```python
from build123d import *

# Parameters (mm, degrees)
BOSS_EXTRUDE1_DEPTH = 17.78
SKETCH2_R           = 2.286
CUT_EXTRUDE1_DEPTH  = 36.070400967
SKETCH3_R           = 2.286
SKETCH3_R_2         = 4.572
CUT_EXTRUDE2_DEPTH  = 2.54
FILLET1_R           = 1.016
FILLET2_R           = 2.54


with BuildPart() as part:
    # Sketch1 → Boss-Extrude1 (new body)
    with BuildSketch(Plane(origin=(0, 0, 0), x_dir=(0, 0, -1), z_dir=(1, 0, 0))):
        Polygon((0, 0), (0, 27.432), (-12.7, 27.432), (-12.7, 15.24), (-3.556, 15.24), (-3.556, 0), align=None)
    extrude(amount=BOSS_EXTRUDE1_DEPTH)

    # Sketch2 → Cut-Extrude1 (cut, through all)
    with BuildSketch(Plane.XY.offset(12.7)):
        with Locations((4.445, 21.082)):
            Circle(SKETCH2_R)
        with Locations(Location((13.335, 21.082, 0), (0, 0, 180))):
            Circle(SKETCH2_R)
    extrude(amount=-CUT_EXTRUDE1_DEPTH, mode=Mode.SUBTRACT)

    # Sketch3 → Cut-Extrude2 (cut)
    # profile 1 of 4: a face of its own
    with BuildSketch(Plane.XY.offset(12.7)):
        with BuildLine():
            ThreePointArc((8.89, 20.011878979), (8.763, 21.082), (8.89, 22.152121021))
            ThreePointArc((8.89, 22.152121021), (4.445, 25.654), (0, 22.152121021))
            Line((0, 22.152121021), (0, 20.011878979))
            ThreePointArc((0, 20.011878979), (4.445, 16.51), (8.89, 20.011878979))
        make_face()
        with Locations((4.445, 21.082)):
            Circle(SKETCH3_R, mode=Mode.SUBTRACT)
    # profile 2 of 4: a face of its own
    with BuildSketch(Plane.XY.offset(12.7)):
        with BuildLine():
            ThreePointArc((8.89, 22.152121021), (8.985138985, 21.620815367), (9.017, 21.082))
            ThreePointArc((9.017, 21.082), (8.985138985, 20.543184633), (8.89, 20.011878979))
            ThreePointArc((8.89, 20.011878979), (13.335, 16.51), (17.78, 20.011878979))
            Line((17.78, 20.011878979), (17.78, 22.152121021))
            ThreePointArc((17.78, 22.152121021), (13.335, 25.654), (8.89, 22.152121021))
        make_face()
        with Locations((13.335, 21.082)):
            Circle(SKETCH3_R, mode=Mode.SUBTRACT)
    # profile 3 of 4: a face of its own
    with BuildSketch(Plane.XY.offset(12.7)):
        with Locations((4.445, 21.082)):
            Circle(SKETCH3_R_2)
    # profile 4 of 4: a face of its own
    with BuildSketch(Plane.XY.offset(12.7)):
        with Locations((13.335, 21.082)):
            Circle(SKETCH3_R_2)
    extrude(amount=-CUT_EXTRUDE2_DEPTH, mode=Mode.SUBTRACT)

    # Fillet1
    fillet1_edges = [part.edges().sort_by_distance(p)[0] for p in [
        (17.78, 15.24, 8.128),
        (8.89, 20.011878979, 11.43),
        (0, 20.011878979, 11.43),
        (0, 22.152121021, 11.43),
        (8.89, 22.152121021, 11.43),
        (17.78, 22.152121021, 11.43),
        (17.78, 20.011878979, 11.43),
        (0, 15.24, 8.128),
    ]]
    fillet(fillet1_edges, radius=FILLET1_R)

    # Fillet2
    # the kernel refuses this fillet: 2.54 mm, written as the material it takes off along each edge
    with BuildSketch(Plane(origin=(0, 27.432, -6.35), x_dir=(0, -1, 0), z_dir=(0, 0, 1))) as fillet2_piece_1:
        with BuildLine():
            CenterArc((FILLET2_R, FILLET2_R), FILLET2_R, 180, 90)
            Line((0, FILLET2_R), (-FILLET2_R * 0.02, FILLET2_R))
            Line((-FILLET2_R * 0.02, FILLET2_R), (-FILLET2_R * 0.02, -FILLET2_R * 0.02))
            Line((-FILLET2_R * 0.02, -FILLET2_R * 0.02), (FILLET2_R, -FILLET2_R * 0.02))
            Line((FILLET2_R, -FILLET2_R * 0.02), (FILLET2_R, 0))
        make_face()
    extrude(amount=25.4, mode=Mode.SUBTRACT)
    with BuildSketch(Plane(origin=(17.78, 27.432, -6.35), x_dir=(0, -1, 0), z_dir=(0, 0, 1))) as fillet2_piece_2:
        with BuildLine():
            CenterArc((FILLET2_R, -FILLET2_R), FILLET2_R, 90, 90)
            Line((0, -FILLET2_R), (-FILLET2_R * 0.02, -FILLET2_R))
            Line((-FILLET2_R * 0.02, -FILLET2_R), (-FILLET2_R * 0.02, FILLET2_R * 0.02))
            Line((-FILLET2_R * 0.02, FILLET2_R * 0.02), (FILLET2_R, FILLET2_R * 0.02))
            Line((FILLET2_R, FILLET2_R * 0.02), (FILLET2_R, 0))
        make_face()
    extrude(amount=25.4, mode=Mode.SUBTRACT)
    with BuildSketch(Plane(origin=(0, 0, 9.906), x_dir=(0, 1, 0), z_dir=(0, 0, -1))) as fillet2_piece_3:
        with BuildLine():
            CenterArc((FILLET2_R, FILLET2_R), FILLET2_R, 180, 90)
            Line((0, FILLET2_R), (-FILLET2_R * 0.02, FILLET2_R))
            Line((-FILLET2_R * 0.02, FILLET2_R), (-FILLET2_R * 0.02, -FILLET2_R * 0.02))
            Line((-FILLET2_R * 0.02, -FILLET2_R * 0.02), (FILLET2_R, -FILLET2_R * 0.02))
            Line((FILLET2_R, -FILLET2_R * 0.02), (FILLET2_R, 0))
        make_face()
    extrude(amount=16.256, mode=Mode.SUBTRACT)
    with BuildSketch(Plane(origin=(17.78, 0, 9.906), x_dir=(0, 1, 0), z_dir=(0, 0, -1))) as fillet2_piece_4:
        with BuildLine():
            CenterArc((FILLET2_R, -FILLET2_R), FILLET2_R, 90, 90)
            Line((0, -FILLET2_R), (-FILLET2_R * 0.02, -FILLET2_R))
            Line((-FILLET2_R * 0.02, -FILLET2_R), (-FILLET2_R * 0.02, FILLET2_R * 0.02))
            Line((-FILLET2_R * 0.02, FILLET2_R * 0.02), (FILLET2_R, FILLET2_R * 0.02))
            Line((FILLET2_R, FILLET2_R * 0.02), (FILLET2_R, 0))
        make_face()
    extrude(amount=16.256, mode=Mode.SUBTRACT)


solid = part.part
```
Geometry check sheet. Reference: the model listing, model coordinates, mm. A direction names the side the tool comes from. Round coordinates to 2 decimals unless told otherwise and drop trailing zeros. Write each loop counter-clockwise with the first axis right and the second up, starting at its lowest first coordinate (ties: lowest second). Pieces come first, ordered by that corner, then holes. Notation, with made-up numbers: (75.25, 65.25) - (82.25, 65.25) arc R31 ccw to (82.25, 95.25) - close; hole circle Ø11 at (48, 25). An arc over 180 degrees is marked (long way). Write each question's results on one line, items separated by ' | '.
(1) Set-up check for faces 1 (the face through (0.69, 24.53, 11.41)), 2 (the face through (17.474, 15.53, 8.064)), 3 (the face through (9, 27.432, 6)), 4 (the face through (0.306, 15.53, 8.064)): record each of +Z, -Z, +X, -X, +Y, -Y from which the full face is reachable in a straight line by a thin tool's end or side.
Computed:
face 1: +Z | face 2: +Z, +X, -Y | face 3: +Z, -Z, +X, -X, +Y | face 4: +Z, -X, -Y
(2) Draft check along Y on faces 5 (the face through (15.02, 19.54, 5.15)), 6 (the face through (9, 8, 3.556)), 7 (the face through (4.985, 16.542, 11.448)), 8 (the face through (0.764, 0.724, 1.803)). Enter one of: pulls with the +Y half, pulls with the -Y half, needs draft (parallel to the pull), parting line crosses it, or undercut.
Computed:
face 5: undercut | face 6: needs draft | face 7: undercut | face 8: pulls with the -Y half
(3) Sectioned sample at C-C, the plane z = 2.5. Enter the section's corners in (x, y) (3 decimals).
Computed:
outline: (0, 2.54) arc R2.54 ccw to (2.54, 0) - (15.24, 0) arc R2.54 ccw to (17.78, 2.54) - (17.78, 24.892) arc R2.54 ccw to (15.24, 27.432) - (2.54, 27.432) arc R2.54 ccw to (0, 24.892) - close; hole circle Ø4.572 at (4.445, 21.082); hole circle Ø4.572 at (13.335, 21.082)
(4) Sectioned sample at A-A, the plane y = 22. Enter the section's corners in (x, z), plus the area to 3 significant figures.
Computed:
outline: (0, 0) - (2.35, 0) - (2.35, 10.16) - (0, 10.16) - close; (6.54, 0) - (11.24, 0) - (11.24, 10.16) - (6.54, 10.16) - close; (15.43, 0) - (17.78, 0) - (17.78, 10.16) - (15.43, 10.16) - close | area: 95.6 mm^2
(5) Sectioned sample at D-D, the plane y = 18. Enter the section's corners in (x, z).
Computed:
outline: (0, 0) - (17.78, 0) - (17.78, 10.16) - (9.96, 10.16) - (9.96, 12.7) - (7.82, 12.7) - (7.82, 10.16) - (0, 10.16) - close
(6) Thickness scan on probe 1 along Z at (x, y) = (2.25, 22.75); probe 2 along X at (y, z) = (16, 10); probe 3 along Y at (x, z) = (2.25, 10.75). Record the ranges inside material, lowest first. Write a range as from..to.
Computed:
probe 1: z = 0..10.16 | probe 2: x = 0.03..17.75 | probe 3: y = 15.24..17.07, 25.09..27.42
(7) Depth check by flat-ended pin: pin 1 Ø4 at (x, y) = (13, 8.5) entering from +Z. Enter the tip coordinate at first touch or a pass-through.
Computed:
pin 1: stops at z = 3.56
(8) Sectioned sample at B-B, the plane x = 12. Enter the section's corners in (y, z), plus the area to 3 significant figures.
Computed:
outline: (0, 0) - (19.23, 0) - (19.23, 10.16) - (16.71, 10.16) - (16.71, 12.7) - (15.24, 12.7) - (15.24, 3.56) - (0, 3.56) - close; (22.94, 0) - (27.43, 0) - (27.43, 12.7) - (25.45, 12.7) - (25.45, 10.16) - (22.94, 10.16) - close | area: 149 mm^2
